Part model, mm, in its own coordinate system. Face numbers are marked on the shaded views. A direction names the side the tool comes from. Round coordinates to 2 decimals unless told otherwise and drop trailing zeros. Write each loop counter-clockwise with the first axis right and the second up, starting at its lowest first coordinate (ties: lowest second). Pieces come first, ordered by that corner, then holes. Notation, with made-up numbers: (28, 48.5) -> (72, 48.5) arc R27 cw to (72, 87.5) -> close; hole circle Ø8 at (-20.5, -7.5). An arc over 180 degrees is marked (long way). Return JSON: item names as keys, results as strings. Group by question number.
(1) Saw through at B-B (z = 0.35). State how many separate pieces and enclosed holes the cut face has, plus the area to 3 significant figures.
(2) Drop flat-ended pins along their axis: pin 1 Ø2 at (x, z) = (-6, 1) entering from -Y; pin 2 Ø9 at (x, y) = (0, 0) entering from -Z; pin 3 Ø1.5 at (y, z) = (2, 0) entering from -X. Give the stop position or say it passes through.
(3) Saw through at D-D (z = -2.25). List the corners of the cut face in (x, y).
(4) Mould opens along X. For the marked faces 6, 7 and 8 say: +X half, -X half, draft (parallel to the pull), parting line (faces both ways), or undercut.
(5) Drill centre lines: L1, parallel to Y at x = 0, z = -2; L2, parallel to Y at x = -5.75, z = 1.35. Where is each one in solid material? Low to high. Write a range as from..to.
(6) Saw through at A-A (y = 0). List the corners of the cut face in (x, z).
(7) Tool access for the marked faces 1, 2, 3, 4 and 5: list every direction of +Z, -Z, +X, -X, +Y, -Y with a clear straight run to the whole face (end or side of a thin tool).
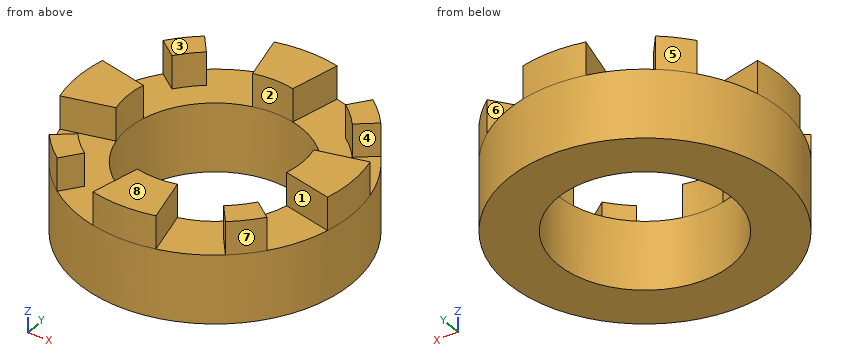
from build123d import *

# Parameters (mm, degrees)
F1_DEPTH = 1.9
F2_DEPTH = 1.9
F3_COUNT = 4
F4_R     = 7.85
F4_R_2   = 5
F6_DEPTH = 3.93


with BuildPart() as f1:
    # F0 (on Top) → F1 (new body)
    with BuildSketch(Plane.XY):
        with BuildLine():
            Line((1.146497, 4.86678), (1.8, 7.640844))
            ThreePointArc((1.8, 7.640844), (0, 7.85), (-1.8, 7.640844))
            Line((-1.8, 7.640844), (-1.146497, 4.86678))
            ThreePointArc((-1.146497, 4.86678), (0, 5), (1.146497, 4.86678))
        make_face()
    extrude(amount=F1_DEPTH)



with BuildPart() as f2:
    # F0 (on Top) → F2 (new body, through all)
    with BuildSketch(Plane.XY):
        with BuildLine():
            ThreePointArc((3.973246, 5.144251), (4.596194, 4.596194), (5.144251, 3.973246))
            Line((5.144251, 3.973246), (6.212672, 4.798459))
            ThreePointArc((6.212672, 4.798459), (5.550788, 5.550788), (4.798459, 6.212672))
            Line((4.798459, 6.212672), (3.973246, 5.144251))
        make_face()
    extrude(amount=F2_DEPTH)


with BuildPart() as f3_1:
    # F3: instance of F1
    add(f1.part.rotate(Axis((0, 0, 0), (0, 0, -1)), 1 * 360 / F3_COUNT))


with BuildPart() as f3_2:
    # F3: instance of F1
    add(f1.part.rotate(Axis((0, 0, 0), (0, 0, -1)), 2 * 360 / F3_COUNT))


with BuildPart() as f3_3:
    # F3: instance of F1
    add(f1.part.rotate(Axis((0, 0, 0), (0, 0, -1)), 3 * 360 / F3_COUNT))


with BuildPart() as f3_4:
    # F3: instance of F2
    add(f2.part.rotate(Axis((0, 0, 0), (0, 0, -1)), 1 * 360 / F3_COUNT))


with BuildPart() as f3_5:
    # F3: instance of F2
    add(f2.part.rotate(Axis((0, 0, 0), (0, 0, -1)), 2 * 360 / F3_COUNT))


with BuildPart() as f3_6:
    # F3: instance of F2
    add(f2.part.rotate(Axis((0, 0, 0), (0, 0, -1)), 3 * 360 / F3_COUNT))


with BuildPart() as f1_1:
    add(f1.part)

    add(f2.part)  # F6 merges F2

    add(f3_1.part)  # F6 merges F3_1

    add(f3_2.part)  # F6 merges F3_2

    add(f3_3.part)  # F6 merges F3_3

    add(f3_4.part)  # F6 merges F3_4

    add(f3_5.part)  # F6 merges F3_5

    add(f3_6.part)  # F6 merges F3_6
    # F4 (on Top) → F6 (join)
    with BuildSketch(Plane.XY):
        Circle(F4_R)
        Circle(F4_R_2, mode=Mode.SUBTRACT)
    extrude(amount=-F6_DEPTH)


solid = f1_1.part
Computed values:
{
 "1": {"separate pieces": "8", "enclosed holes": "0", "area": "43.8 mm2"},
 "2": {"pin 1": "y = -6.05", "pin 2": "through", "pin 3": "x = -7.75"},
 "3": {"outline": "circle Ø15.7 at (0, 0); hole circle Ø10 at (0, 0)"},
 "4": {"face 6": "undercut", "face 7": "+X half", "face 8": "draft"},
 "5": {"L1": "-7.85..-5, 5..7.85", "L2": "-5.34..-4.44, -1.35..1.35, 4.44..5.34"},
 "6": {"outline": "(-7.85, -3.93) -> (-5, -3.93) -> (-5, 1.9) -> (-7.85, 1.9) -> close; (5, -3.93) -> (7.85, -3.93) -> (7.85, 1.9) -> (5, 1.9) -> close"},
 "7": {"face 1": "+Z", "face 2": "+Z, -Z", "face 3": "+Z, +X, -X, +Y, -Y", "face 4": "+Z, +X", "face 5": "+Z, -Z, -X, +Y"}
}
